The model under review builds one solid part; all positions refer to its coordinate system, in mm. Face numbers are marked on the shaded views. Round coordinates to 2 decimals unless told otherwise and drop trailing zeros. Order: outer loops, then holes, each group sorted by start corner. A loop starts at its lowest first (then second) coordinate and runs counter-clockwise, first axis right, second up. Notation, with made-up numbers: M 61.5,83 L 69.5,83 A16 cw 69.5,90 Z; hole C 55.5,65 d3. An arc over 180 degrees is marked long. Answer as a JSON object with one key per item and string values. Group by question number.
1. Clearance check with flat-ended pins moving along their axes: P1, Ø10, axis at y = 25, z = 11.5, coming from the +X side; P2, Ø8, axis at x = 19.5, z = 15.5, coming from the -Y side; P3, Ø2, axis at y = 52, z = -14, coming from the -X side; P4, Ø1, axis at x = 18.5, y = 5, coming from the +Z side. State where each tip first meets the part, or that it passes through.
2. Add section B-B on x = 0. State the section outline as (y, z) points.
3. To check wall thickness, follow probe 1 along Z at (x, y) = (0, -6); probe 2 along Z at (x, y) = (-17.5, 25); probe 3 along X at (y, z) = (54, 13). State the ranges of each line that lie inside material, in increasing order. Write a range as [from, to].
4. Add section A-A on z = 0. State the section outline as (x, y) points.
5. Add section C-C on y = 48. State the section outline as (x, z) points.
6. Add section D-D on z = 20. State the section outline as (x, y) points, and give its area (3 significant figures).
7. Mouldability with a two-part tool opening along Z and no side actions: class the marked faces 1 and 2 as released by +Z, released by -Z, zero draft, split by the parting line, or undercut.
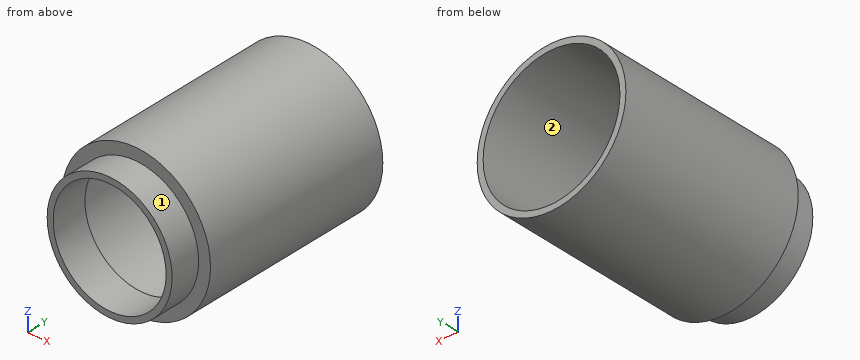
Autodesk Inventor part; units mm, degrees
ref_plane "YZ Plane" through (0, 0, 0) normal (1, 0, 0) x (0, 1, 0)
ref_plane "XZ Plane" through (0, 0, 0) normal (0, 1, 0) x (-1, 0, 0)
ref_plane "XY Plane" through (0, 0, 0) normal (0, 0, 1) x (1, 0, 0)
sketch "Sketch1" plane through (0, 0, 0) normal (0, 0, 1) x (1, 0, 0)
  line L0 (0, 0) -> (25, 0) construction
  line L1 (25, 0) -> (25, 65) construction
  line L2 (25, 65) -> (0, 65) construction
  line L3 (0, 65) -> (0, 0) construction
  line L4 (25, 65) -> (23, 65)
  line L5 (23, 65) -> (23, 0)
  line L6 (23, 0) -> (25, 0)
  line L7 (25, 0) -> (25, 65)
  line L8 (0, 0) -> (21, 0) construction
  line L9 (21, 0) -> (21, -10) construction
  line L10 (21, -10) -> (0, -10) construction
  line L11 (0, -10) -> (0, 0) construction
  line L12 (21, 0) -> (19, 0)
  line L13 (19, 0) -> (19, -10)
  line L14 (19, -10) -> (21, -10)
  line L15 (21, -10) -> (21, 0)
  line L16 (19, 0) -> (25, 0)
  line L17 (25, 0) -> (25, 2)
  line L18 (25, 2) -> (19, 2)
  line L19 (19, 2) -> (19, 0)
  point P0 (23, 2)
  dimension "d0" = 25
  dimension "d1" = 65
  dimension "d2" = 2
  dimension "d3" = 21
  dimension "d4" = 10
  dimension "d5" = 2
  dimension "d6" = 2
revolve "Revolution1" add sketch "Sketch1" angle 360 about axis through (0, 65, 0) along (0, -1, 0)
properties part number "flour_duct"
Recorded:
{
 "1": {"P1": "stops at x = 24.14", "P2": "stops at y = -10", "P3": "stops at x = -21.35", "P4": "stops at z = 17.35"},
 "2": {"outline": "M -10,-21 L 0,-21 L 0,-25 L 65,-25 L 65,-23 L 2,-23 L 2,-19 L -10,-19 Z; M -10,19 L 2,19 L 2,23 L 65,23 L 65,25 L 0,25 L 0,21 L -10,21 Z"},
 "3": {"probe 1": "z = [-21, -19], [19, 21]", "probe 2": "z = [-17.85, -14.92], [14.92, 17.85]", "probe 3": "x = [-21.35, -18.97], [18.97, 21.35]"},
 "4": {"outline": "M -25,0 L -21,0 L -21,-10 L -19,-10 L -19,2 L -23,2 L -23,65 L -25,65 Z; M 19,-10 L 21,-10 L 21,0 L 25,0 L 25,65 L 23,65 L 23,2 L 19,2 Z"},
 "5": {"outline": "C 0,0 d50; hole C 0,0 d46"},
 "6": {"outline": "M -15,0 L -6.4,0 L -6.4,-10 L 6.4,-10 L 6.4,0 L 15,0 L 15,65 L 11.36,65 L 11.36,2 L -11.36,2 L -11.36,65 L -15,65 Z", "area": "647 mm²"},
 "7": {"face 1": "split by the parting line", "face 2": "undercut"}
}
